The model under review builds one solid part; all positions refer to its coordinate system, in mm. Coordinates: 2 decimals unless noted, no trailing zeros. Loops run counter-clockwise (first coordinate to the right, second up) from the corner with the lowest first, then second, coordinate; pieces in that order, holes last. Notation, with made-up numbers: M 38.5,-23 L 49.5,-23 A17 cw 49.5,10 Z; hole C 77.5,57 d2. An arc over 180 degrees is marked long. Write item = value, one per line. Start each with the question number.
Q1. Mouldability with a two-part tool opening along X and no side actions: class faces 1 (the face through (-28.19, -1, -22)), 2 (the face through (8.82, -0.74, -10.94)), 3 (the face through (63.369, -1, -22)), 4 (the face through (18, -1.5, -15)) as released by +X, released by -X, zero draft, split by the parting line, or undercut.
Q2. We need section A-A on x = -10. Give the boundary of the cut face in (y, z), and give its area (4 significant figures).
Q3. We need section C-C on y = -0.95. Count the separate pieces of the cut face and the enclosed holes in it, and give its area (3 significant figures).
Q4. Wall thickness on probe 1 along Z at (x, y) = (-20, -1.05); probe 2 along X at (y, z) = (-1.15, -1.5); probe 3 along Z at (x, y) = (51, -0.4): over which ranges is each line inside the solid? List them lowest first.
Q5. We need section D-D on x = -19.5. Give the boundary of the cut face in (y, z), and give its area (3 significant figures).
Q6. We need section B-B on z = -20. Give the boundary of the cut face in (x, y).
Autodesk Inventor part; units mm, degrees
ref_plane "YZ Plane" through (0, 0, 0) normal (1, 0, 0) x (0, 1, 0)
ref_plane "XZ Plane" through (0, 0, 0) normal (0, 1, 0) x (-1, 0, 0)
ref_plane "XY Plane" through (0, 0, 0) normal (0, 0, 1) x (1, 0, 0)
sketch "Sketch1" plane through (0, 0, 0) normal (0, 1, 0) x (-1, 0, 0)
  line L0 (-0.4496, -30) -> (-0.4496, 0)
  line L1 (-34.7289, 0) -> (-34.7289, -30)
  circle A0 centre (-45.1786, -20) radius 1.55
  circle A1 centre (10, -20) radius 1.55
  circle A2 centre (-55.1786, -20) radius 1.55
  circle A3 centre (20, -20) radius 1.55
  circle A4 centre (-27.5893, -10) radius 1.55
  circle A5 centre (-27.5893, -20) radius 1.55
  circle A6 centre (-7.5893, -10) radius 1.55
  circle A7 centre (-7.5893, -20) radius 1.55
  arc A8 (13.7758, -0.5858) -> (12.3616, 0) centre (12.3616, -2) ccw
  line L2 (27.6042, -14.4142) -> (13.7758, -0.5858)
  arc A9 (28.19, -15.8284) -> (27.6042, -14.4142) centre (26.19, -15.8284) ccw
  line L3 (28.19, -15.8284) -> (28.19, -28)
  arc A10 (26.19, -30) -> (28.19, -28) centre (26.19, -28) ccw
  arc A11 (-47.5401, 0) -> (-48.9543, -0.5858) centre (-47.5401, -2) ccw
  line L4 (-48.9543, -0.5858) -> (-62.7828, -14.4142)
  arc A12 (-62.7828, -14.4142) -> (-63.3686, -15.8284) centre (-61.3686, -15.8284) ccw
  line L5 (-63.3686, -28) -> (-63.3686, -15.8284)
  arc A13 (-63.3686, -28) -> (-61.3686, -30) centre (-61.3686, -28) ccw
  line L6 (-47.5401, 0) -> (12.3616, 0)
  line L7 (26.19, -30) -> (-61.3686, -30)
  line L8 (-35.1786, -30) -> (-35.1786, 0)
  line L9 (-34.2793, 0) -> (-34.2793, -30)
  line L10 (-0.8993, -30) -> (-0.8993, 0)
  line L11 (0, 0) -> (0, -30)
extrude "Extrusion1" add sketch "Sketch1" against normal blind 1.5
properties part number "Head1"
Returned:
q1.face_1 = released by -X
q1.face_2 = undercut
q1.face_3 = released by +X
q1.face_4 = zero draft
q2.outline = M -1.5,-30 L 0,-30 L 0,-21.55 L -1.5,-21.55 Z; M -1.5,-18.45 L 0,-18.45 L 0,0 L -1.5,0 Z
q2.area = 40.35 mm^2
q3.separate_pieces = 1
q3.enclosed_holes = 8
q3.area = 2,460 mm^2
q4.probe_1 = -30 to -21.55, -18.45 to -6.81
q4.probe_2 = -14.69 to 49.87
q4.probe_3 = -30 to -2.63
q5.outline = M -1.5,-30 L 0,-30 L 0,-21.47 L -1.5,-21.47 Z; M -1.5,-18.53 L 0,-18.53 L 0,-6.31 L -1.5,-6.31 Z
q5.area = 31.1 mm^2
q6.outline = M -28.19,-1.5 L -21.55,-1.5 L -21.55,0 L -28.19,0 Z; M -18.45,-1.5 L -11.55,-1.5 L -11.55,0 L -18.45,0 Z; M -8.45,-1.5 L 6.04,-1.5 L 6.04,0 L -8.45,0 Z; M 9.14,-1.5 L 26.04,-1.5 L 26.04,0 L 9.14,0 Z; M 29.14,-1.5 L 43.63,-1.5 L 43.63,0 L 29.14,0 Z; M 46.73,-1.5 L 53.63,-1.5 L 53.63,0 L 46.73,0 Z; M 56.73,-1.5 L 63.37,-1.5 L 63.37,0 L 56.73,0 Z
